Geometry check sheet. Reference: the model listing, model coordinates, mm. A direction names the side the tool comes from. Coordinates: 2 decimals unless noted, no trailing zeros. Order: outer loops, then holes, each group sorted by start corner. A loop starts at its lowest first (then second) coordinate and runs counter-clockwise, first axis right, second up. Notation, with made-up numbers: (81.5, 27) - (107.5, 27) arc R13 ccw to (107.5, 48) - close; hole circle Ø7 at (50.25, 17). An arc over 180 degrees is marked (long way). Put each result on its own line as item: value.
from build123d import *

# Parameters (mm, degrees)
BOSS_EXTRUDE1_DEPTH = 3.175


with BuildPart() as part:
    # Sketch1 → Boss-Extrude1 (new body)
    with BuildSketch(Plane.XY):
        with BuildLine():
            Line((-8.1, 0), (8.1, 0))
            Line((8.1, 0), (10.75, -2.65))
            Line((10.75, -2.65), (10.75, -3.65))
            Line((10.75, -3.65), (4.2, -3.65))
            ThreePointArc((4.2, -3.65), (2.550037108, -5.288934004), (4.177868505, -6.949851568))
            ThreePointArc((4.177868505, -6.949851568), (47.407650937, -20.329895347), (76.461639413, -55.024353322))
            ThreePointArc((76.461639413, -55.024353322), (86.688165284, -58.25355516), (89.960911147, -68.466229169))
            ThreePointArc((89.960911147, -68.466229169), (86.704969014, -70.755892654), (84.44942629, -67.476221165))
            ThreePointArc((84.44942629, -67.476221165), (81.554604124, -62.18029995), (75.8, -64))
            Line((75.8, -64), (81.646374133, -70.967437377))
            Line((81.646374133, -70.967437377), (96.044354863, -124.701432988))
            ThreePointArc((96.044354863, -124.701432988), (96.437025669, -125.261990951), (97.098218064, -125.438739948))
            ThreePointArc((97.098218064, -125.438739948), (104.73060086, -128.02457671), (107.977591805, -135.4))
            ThreePointArc((107.977591805, -135.4), (105.477591805, -137.9), (102.977591805, -135.4))
            ThreePointArc((102.977591805, -135.4), (101.386328057, -132.386015089), (98, -132))
            Line((98, -132), (117.691047305, -205.487988996))
            ThreePointArc((117.691047305, -205.487988996), (120.056868172, -206.85389631), (121.422775486, -204.488075443))
            Line((121.422775486, -204.488075443), (120.128680261, -199.658446312))
            ThreePointArc((120.128680261, -199.658446312), (122.250000605, -195.984211697), (125.924235219, -198.105532041))
            Line((125.924235219, -198.105532041), (127.218330444, -202.935161172))
            ThreePointArc((127.218330444, -202.935161172), (121.609782443, -212.649451268), (111.895492347, -207.040903266))
            Line((111.895492347, -207.040903266), (84.010461962, -102.9725531))
            ThreePointArc((84.010461962, -102.9725531), (83.826764804, -102.418590939), (83.579767988, -101.889808095))
            ThreePointArc((83.579767988, -101.889808095), (71.468601459, -84.461922175), (55.79064441, -70.157614254))
            ThreePointArc((55.79064441, -70.157614254), (54.487597498, -68.761604863), (53.802955351, -66.978899446))
            Line((53.802955351, -66.978899446), (48.2152775, -35.289603638))
            ThreePointArc((48.2152775, -35.289603638), (47.508195964, -33.471346485), (46.159120917, -32.062084305))
            Line((46.159120917, -32.062084305), (38.847152873, -26.942189162))
            ThreePointArc((38.847152873, -26.942189162), (36.061695911, -27.433340377), (36.552847127, -30.218797339))
            Line((36.552847127, -30.218797339), (41.349143695, -33.577200351))
            ThreePointArc((41.349143695, -33.577200351), (42.698218742, -34.986462531), (43.405300278, -36.804719684))
            Line((43.405300278, -36.804719684), (47.924038765, -62.431759112))
            ThreePointArc((47.924038765, -62.431759112), (45.976650255, -67.317406285), (40.735673212, -67.757894593))
            ThreePointArc((40.735673212, -67.757894593), (20.943431619, -60.476046738), (0, -58))
            ThreePointArc((0, -58), (-20.943431619, -60.476046738), (-40.735673212, -67.757894593))
            ThreePointArc((-40.735673212, -67.757894593), (-45.976650255, -67.317406285), (-47.924038765, -62.431759112))
            Line((-47.924038765, -62.431759112), (-43.405300278, -36.804719684))
            ThreePointArc((-43.405300278, -36.804719684), (-42.698218742, -34.986462531), (-41.349143695, -33.577200351))
            Line((-41.349143695, -33.577200351), (-36.552847127, -30.218797339))
            ThreePointArc((-36.552847127, -30.218797339), (-36.061695911, -27.433340377), (-38.847152873, -26.942189162))
            Line((-38.847152873, -26.942189162), (-46.159120917, -32.062084305))
            ThreePointArc((-46.159120917, -32.062084305), (-47.508195964, -33.471346485), (-48.2152775, -35.289603638))
            Line((-48.2152775, -35.289603638), (-53.802955351, -66.978899446))
            ThreePointArc((-53.802955351, -66.978899446), (-54.487597498, -68.761604863), (-55.79064441, -70.157614254))
            ThreePointArc((-55.79064441, -70.157614254), (-71.468601459, -84.461922175), (-83.579767988, -101.889808095))
            ThreePointArc((-83.579767988, -101.889808095), (-83.826764804, -102.418590939), (-84.010461962, -102.9725531))
            Line((-84.010461962, -102.9725531), (-111.895492347, -207.040903266))
            ThreePointArc((-111.895492347, -207.040903266), (-121.609782443, -212.649451268), (-127.218330444, -202.935161172))
            Line((-127.218330444, -202.935161172), (-125.924235219, -198.105532041))
            ThreePointArc((-125.924235219, -198.105532041), (-122.250000605, -195.984211697), (-120.128680261, -199.658446312))
            Line((-120.128680261, -199.658446312), (-121.422775486, -204.488075443))
            ThreePointArc((-121.422775486, -204.488075443), (-120.056868172, -206.85389631), (-117.691047305, -205.487988996))
            Line((-117.691047305, -205.487988996), (-98, -132))
            ThreePointArc((-98, -132), (-101.386328057, -132.386015089), (-102.977591805, -135.4))
            ThreePointArc((-102.977591805, -135.4), (-105.477591805, -137.9), (-107.977591805, -135.4))
            ThreePointArc((-107.977591805, -135.4), (-104.73060086, -128.02457671), (-97.098218064, -125.438739948))
            ThreePointArc((-97.098218064, -125.438739948), (-96.437025669, -125.261990951), (-96.044354863, -124.701432988))
            Line((-96.044354863, -124.701432988), (-81.646374133, -70.967437377))
            Line((-81.646374133, -70.967437377), (-75.8, -64))
            ThreePointArc((-75.8, -64), (-81.554604124, -62.18029995), (-84.44942629, -67.476221165))
            ThreePointArc((-84.44942629, -67.476221165), (-86.704969014, -70.755892654), (-89.960911147, -68.466229169))
            ThreePointArc((-89.960911147, -68.466229169), (-86.688165284, -58.25355516), (-76.461639413, -55.024353322))
            ThreePointArc((-76.461639413, -55.024353322), (-47.407650937, -20.329895347), (-4.177868505, -6.949851568))
            ThreePointArc((-4.177868505, -6.949851568), (-2.550037108, -5.288934004), (-4.2, -3.65))
            Line((-4.2, -3.65), (-10.75, -3.65))
            Line((-10.75, -3.65), (-10.75, -2.65))
            Line((-10.75, -2.65), (-8.1, 0))
        make_face()
    extrude(amount=BOSS_EXTRUDE1_DEPTH)


solid = part.part
Q1. Section check A-A on x = -87.2. Record the boundary of the cut face in (y, z) (3 decimals).
Answer block:
outline: (-114.876, 0) - (-91.694, 0) - (-91.694, 3.175) - (-114.876, 3.175) - close; (-70.8, 0) - (-58.797, 0) - (-58.797, 3.175) - (-70.8, 3.175) - close
Q2. Thickness scan on L1, parallel to X at y = -44, z = 1.55; L2, parallel to X at y = -48.5, z = 2.55; L3, parallel to X at y = -169.5, z = 0.5. Record the ranges inside material, lowest first. Write a range as [from, to].
Answer block:
L1: x = [-70.6, -49.75], [-44.67, 44.67], [49.75, 70.6]
L2: x = [-73.26, -50.54], [-45.47, 45.47], [50.54, 73.26]
L3: x = [-108.05, -101.84], [101.84, 108.05]
Q3. Draft check along X on faces 1 (the flat face through (107.7, -168.2, 1.6)), 2 (the cylindrical face through (-121.441, -212.693, 1.565)), 3 (the flat face through (1, -51, 3.175)), 4 (the flat face through (88.745, -97.458, 1.565)). Enter one of: pulls with the +X half, pulls with the -X half, needs draft (parallel to the pull), parting line crosses it, or undercut.
Answer block:
face 1: undercut
face 2: undercut
face 3: needs draft
face 4: pulls with the +X half
Q4. Access from +Z, -Z, +X, -X, +Y, -Y to the whole of each face (thin tool, end or side, straight path). Record for faces 5 (the flat face through (-88.946, -98.211, 1.565)), 6 (the flat face through (78.68, -67.43, 1.57)), 7 (the cylindrical face through (71.664, -84.686, 1.565)).
Answer block:
face 5: +Z, -Z, -X
face 6: +Z, -Z
face 7: +Z, -Z, -Y
Q5. Section check B-B on y = -83. Record the boundary of the cut face in (x, z) (3 decimals).
Answer block:
outline: (-84.87, 0) - (-70.161, 0) - (-70.161, 3.175) - (-84.87, 3.175) - close; (70.161, 0) - (84.87, 0) - (84.87, 3.175) - (70.161, 3.175) - close
Q6. Section check C-C on x = -22.5. Record the boundary of the cut face in (y, z) (3 decimals).
Answer block:
outline: (-60.864, 0) - (-9.329, 0) - (-9.329, 3.175) - (-60.864, 3.175) - close
Q7. Depth check by flat-ended pin: pin 1 Ø1 at (x, z) = (-6.5, 1) entering from -Y; pin 2 Ø0.8 at (y, z) = (-3, 2) entering from -X; pin 3 Ø1 at (x, z) = (8, 1) entering from -Y. Enter the tip coordinate at first touch or a pass-through.
Answer block:
pin 1: stops at y = -58.27
pin 2: stops at x = -10.75
pin 3: stops at y = -58.4
